Autodesk Inventor part; units mm, degrees
ref_plane "YZ Plane" through (0, 0, 0) normal (1, 0, 0) x (0, 1, 0)
ref_plane "XZ Plane" through (0, 0, 0) normal (0, 1, 0) x (-1, 0, 0)
ref_plane "XY Plane" through (0, 0, 0) normal (0, 0, 1) x (1, 0, 0)
sketch "Sketch1" plane through (0, 0, 0) normal (0, 1, 0) x (-1, 0, 0)
  circle A0 centre (0, 0) radius 11
  dimension "d0" = 22
extrude "Extrusion1" add sketch "Sketch1" along normal blind 6
sketch "Sketch2" plane through (0, 6, 0) normal (0, 1, 0) x (1, 0, 0)
  circle A0 centre (0, 0) radius 8.4
  dimension "d3" = 16.8
extrude "Extrusion2" add sketch "Sketch2" along normal blind 180
sketch "Sketch3" plane through (0, 186, 0) normal (0, 1, 0) x (1, 0, 0)
  circle A0 centre (0, 0) radius 6
  dimension "d6" = 12
extrude "Extrusion3" add sketch "Sketch3" along normal blind 8
fillet "Fillet1" radius 1 2 edges at (11, 0, 0) (11, 6, 0)
fillet "Fillet2" radius 0.5 1 edges at (-8.4, 6, 0)
properties part number "1"
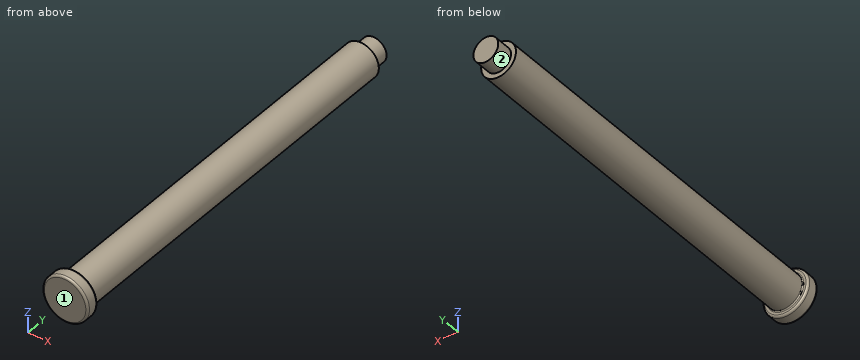
Check sheet for the modelled part. Datum: model origin and axes. Units: mm. Face numbers are marked on the shaded views. A direction names the side the tool comes from. Round coordinates to 2 decimals unless told otherwise and drop trailing zeros. Loops run counter-clockwise (first coordinate to the right, second up) from the corner with the lowest first, then second, coordinate; pieces in that order, holes last. Notation, with made-up numbers: (10, -7.5) -> (43, -7.5) arc R33 ccw to (43, 24.5) -> close; hole circle Ø10 at (60, 8). An arc over 180 degrees is marked (long way). Answer in a Markdown table with one row per item.
Q1. Set-up check for the marked faces 1 and 2: record each of +Z, -Z, +X, -X, +Y, -Y from which the full face is reachable in a straight line by a thin tool's end or side.
Data:
| item | result |
|---|---|
| face 1 | +Z, -Z, +X, -X, -Y |
| face 2 | +Y |
Q2. Sectioned sample at B-B on x = 0. Enter the section's corners in (y, z), then the cut area to 3 significant figures.
Data:
| item | result |
|---|---|
| outline | (0, -10) arc R1 ccw to (1, -11) -> (5, -11) arc R1 ccw to (6, -10) -> (6, -8.9) arc R0.5 cw to (6.5, -8.4) -> (186, -8.4) -> (186, -6) -> (194, -6) -> (194, 6) -> (186, 6) -> (186, 8.4) -> (6.5, 8.4) arc R0.5 cw to (6, 8.9) -> (6, 10) arc R1 ccw to (5, 11) -> (1, 11) arc R1 ccw to (0, 10) -> close |
| area | 3,250 mm^2 |
Q3. Thickness scan on L1, parallel to Z at x = -0.5, y = 152; L2, parallel to Y at x = -8.5, z = 4.5. Record the ranges inside material, lowest first.
Data:
| item | result |
|---|---|
| L1 | z = -8.39 to 8.39 |
| L2 | y = 0 to 6 |
Q4. Sectioned sample at C-C on y = 21.5. Enter the section's corners in (x, z), then the cut area to 3 significant figures.
Data:
| item | result |
|---|---|
| outline | circle Ø16.8 at (0, 0) |
| area | 222 mm^2 |
Q5. Sectioned sample at A-A on z = 0. Enter the section's corners in (x, y).
Data:
| item | result |
|---|---|
| outline | (-11, 1) arc R1 ccw to (-10, 0) -> (10, 0) arc R1 ccw to (11, 1) -> (11, 5) arc R1 ccw to (10, 6) -> (8.9, 6) arc R0.5 cw to (8.4, 6.5) -> (8.4, 186) -> (6, 186) -> (6, 194) -> (-6, 194) -> (-6, 186) -> (-8.4, 186) -> (-8.4, 6.5) arc R0.5 cw to (-8.9, 6) -> (-10, 6) arc R1 ccw to (-11, 5) -> close |
Q6. Go/stop test with flat-tipped pins: P1, Ø3, axis at x = -4, z = -8.5, coming from the +Y side; P2, Ø10, axis at x = -2, y = 121, coming from the +Z side; P3, Ø8, axis at y = 170.5, z = 2, coming from the -X side. Record where each tip stops, or that it passes through.
Data:
| item | result |
|---|---|
| P1 | stops at y = 186 |
| P2 | stops at z = 8.4 |
| P3 | stops at x = -8.4 |
